```python
from build123d import *

# Parameters (mm, degrees)
BOSS_EXTRUDE1_DEPTH = 15
BOSS_EXTRUDE2_DEPTH = 6.33


with BuildPart() as part:
    # Sketch1 → Boss-Extrude1 (new body)
    with BuildSketch(Plane(origin=(0, 0, 87.601912264), x_dir=(-1, 0, 0), z_dir=(0, 0, -1))):
        with BuildLine():
            Line((38.270660543, 36.840565439), (47.370660543, 36.840565439))
            ThreePointArc((47.370660543, 36.840565439), (47.900990629, 36.620895525), (48.120660543, 36.090565439))
            Line((48.120660543, 36.090565439), (48.120660543, 31.090565439))
            ThreePointArc((48.120660543, 31.090565439), (47.900990629, 30.560235353), (47.370660543, 30.340565439))
            Line((47.370660543, 30.340565439), (38.270660543, 30.340565439))
            ThreePointArc((38.270660543, 30.340565439), (37.740330458, 30.560235353), (37.520660543, 31.090565439))
            Line((37.520660543, 31.090565439), (37.520660543, 36.090565439))
            ThreePointArc((37.520660543, 36.090565439), (37.740330458, 36.620895525), (38.270660543, 36.840565439))
        make_face()
    extrude(amount=BOSS_EXTRUDE1_DEPTH)

    # Sketch2 → Boss-Extrude2 (add)
    with BuildSketch(Plane(origin=(0, 0, 72.601912264), x_dir=(-1, 0, 0), z_dir=(0, 0, -1))):
        with BuildLine():
            ThreePointArc((40.320660543, 33.050565439), (39.704827774, 33.289230716), (39.410660543, 33.880565439))
            Line((39.410660543, 33.880565439), (39.410660543, 34.380565439))
            ThreePointArc((39.410660543, 34.380565439), (39.557107153, 34.73411883), (39.910660543, 34.880565439))
            Line((39.910660543, 34.880565439), (45.730660543, 34.880565439))
            ThreePointArc((45.730660543, 34.880565439), (46.084213934, 34.73411883), (46.230660543, 34.380565439))
            Line((46.230660543, 34.380565439), (46.230660543, 33.880565439))
            ThreePointArc((46.230660543, 33.880565439), (45.936493313, 33.289230716), (45.320660543, 33.050565439))
            Line((45.320660543, 33.050565439), (40.320660543, 33.050565439))
        make_face()
    extrude(amount=BOSS_EXTRUDE2_DEPTH)


solid = part.part
```
Design review of the part built by this model. Coordinates are the model's own, in mm. A direction names the side the tool comes from. Coordinates: 2 decimals unless noted, no trailing zeros. Write each loop counter-clockwise with the first axis right and the second up, starting at its lowest first coordinate (ties: lowest second). Pieces come first, ordered by that corner, then holes.
1) Insertion check: pin 1 (4.5 mm diameter, centred on x = -44, z = 71, fed in from +Y); pin 2 (1 mm diameter, centred on y = 33, z = 70.5, fed in from +X); pin 3 (0.6 mm diameter, centred on y = 34, z = 70, fed in from +X); pin 4 (1.5 mm diameter, centred on x = -42.5, z = 68, fed in from -Y). Each pin has a flat end and moves straight along its axis. Give the tip position at first contact, or say it passes through.
2) Add section A-A (x = -41). Write out the cut boundary in (y, z), plus the area to 3 significant figures.
3) Add section C-C (y = 32.75). Write out the cut boundary in (x, z), plus the area to 3 significant figures.
4) Add section D-D (x = -46.75). Write out the cut boundary in (y, z), plus the area to 3 significant figures.
5) Machinability: for faces 1 (the cylindrical face through (-45.943, 33.296, 69.481)), 2 (the cylindrical face through (-39.712, 33.283, 69.481)), 3 (the flat face through (-43, 33.051, 69)), which of the approach directions +Z, -Z, +X, -X, +Y, -Y give a long, thin tool a straight path to every point of the face, cutting with its end or side? Answer none if there is none.
6) Add section B-B (z = 70.5). Write out the cut boundary in (x, y).
7) To check wall thickness, follow L1, parallel to Z at x = -38, y = 32.5; L2, parallel to X at y = 34, z = 72.25; L3, parallel to Y at x = -44, z = 68.75. State the ranges of each line that lie inside material, in increasing order.
Check result:
1. pin 1: stops at y = 36.84
1. pin 2: stops at x = -39.53
1. pin 3: stops at x = -39.41
1. pin 4: stops at y = 33.05
2. outline: (30.34, 72.6) - (33.05, 72.6) - (33.05, 66.27) - (34.88, 66.27) - (34.88, 72.6) - (36.84, 72.6) - (36.84, 87.6) - (30.34, 87.6) - close
2. area: 109 mm2
3. outline: (-48.12, 72.6) - (-37.52, 72.6) - (-37.52, 87.6) - (-48.12, 87.6) - close
3. area: 159 mm2
4. outline: (30.34, 72.6) - (36.84, 72.6) - (36.84, 87.6) - (30.34, 87.6) - close
4. area: 97.5 mm2
5. face 1: -Z, -X, -Y
5. face 2: -Z, +X, -Y
5. face 3: -Z, +X, -X, -Y
6. outline: (-46.23, 33.88) arc R0.91 ccw to (-45.32, 33.05) - (-40.32, 33.05) arc R0.91 ccw to (-39.41, 33.88) - (-39.41, 34.38) arc R0.5 ccw to (-39.91, 34.88) - (-45.73, 34.88) arc R0.5 ccw to (-46.23, 34.38) - close
7. L1: z = 72.6 to 87.6
7. L2: x = -46.23 to -39.41
7. L3: y = 33.05 to 34.88
